Design review of the part shown in the three views and the two pictorial views. Dimensions are in mm from the part's minimum x, y and z. Give positions to 0.01 mm unless a question says otherwise; leave off trailing zeros. Loops run counter-clockwise (first coordinate to the right, second up) from the corner with the lowest first, then second, coordinate; pieces in that order, holes last. Notation, with made-up numbers: (-24.5, -40) -> (-18.5, -40) arc R17 cw to (-18.5, -31) -> close; hole circle Ø6 at (-39.75, -33). An arc over 180 degrees is marked (long way). Answer as CSV lines item,"result". Start each with the question number.
Item 1: Clearance check with flat-ended pins moving along their axes: P1, Ø0.9, axis at x = 67, y = 38.5, coming from the +Z side; P2, Ø2, axis at x = 22.5, y = 48, coming from the +Z side. State where each tip first meets the part, or that it passes through.
Item 2: Add section A-A on y = 8. State the section outline as (x, z) points.
Item 3: The part is to be moulded in two halves that separate along X. For the marked faces 1, 2, 3 and 4, say which applies: +X half, -X half, draft (parallel to the pull), parting line (faces both ways), or undercut.
Item 4: Add section B-B on x = 36.5. State the section outline as (y, z) points.
Item 5: For L1, parallel to X at y = 45, z = 13.75; L2, parallel to X at y = 31, z = 5.75; L3, parallel to Z at x = 28, y = 39, list the stretches that pass through material, from the lowest coordinate up. Write a range as from..to.
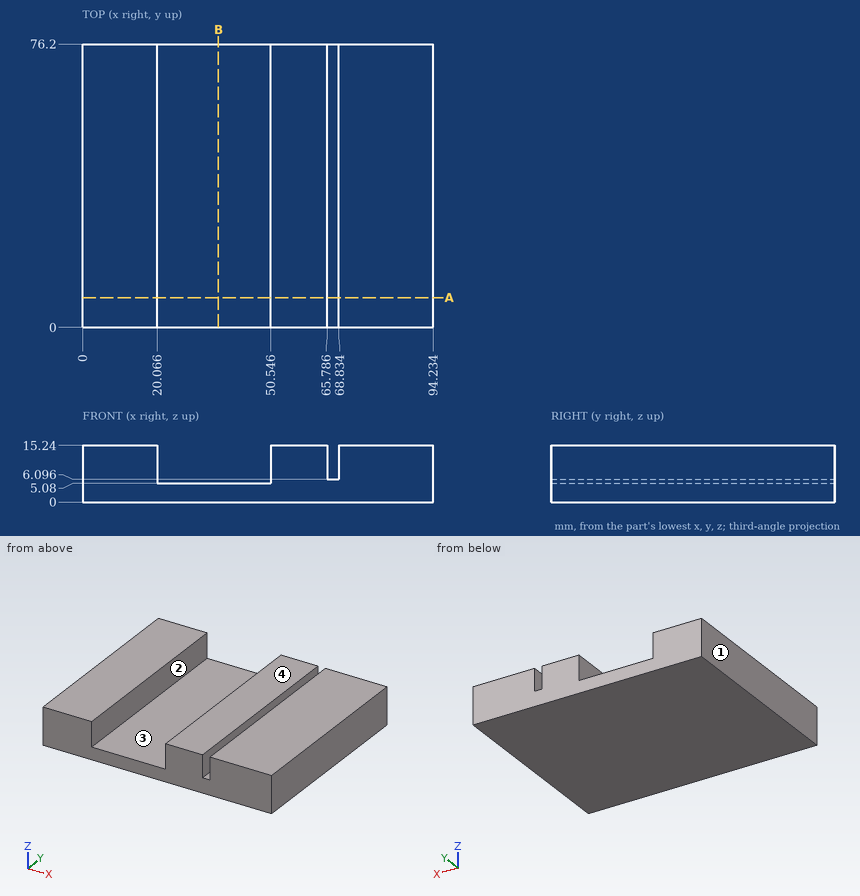
Computed values:
1,P1,"z = 6.1"
1,P2,"z = 5.08"
2,outline,"(0, 0) -> (94.23, 0) -> (94.23, 15.24) -> (68.83, 15.24) -> (68.83, 6.1) -> (65.79, 6.1) -> (65.79, 15.24) -> (50.55, 15.24) -> (50.55, 5.08) -> (20.07, 5.08) -> (20.07, 15.24) -> (0, 15.24) -> close"
3,face 1,"-X half"
3,face 2,"undercut"
3,face 3,"undercut"
3,face 4,"draft"
4,outline,"(0, 0) -> (76.2, 0) -> (76.2, 5.08) -> (0, 5.08) -> close"
5,L1,"0..20.07, 50.55..65.79, 68.83..94.23"
5,L2,"0..20.07, 50.55..94.23"
5,L3,"0..5.08"
